Source: CAD feature listing. Evaluate the final solid. Frame: model axes, mm. A direction names the side the tool comes from. Round coordinates to 2 decimals unless told otherwise and drop trailing zeros. Write each loop counter-clockwise with the first axis right and the second up, starting at its lowest first coordinate (ties: lowest second). Pieces come first, ordered by that corner, then holes. Notation, with made-up numbers: (-27.5, 86) -> (-11.5, 86) arc R20 ccw to (-11.5, 99) -> close; hole circle Ø4 at (74, -40). An arc over 180 degrees is marked (long way). Put each result on its own line as item: value.
Autodesk Inventor part; units mm, degrees
ref_plane "YZ Plane" through (0, 0, 0) normal (1, 0, 0) x (0, 1, 0)
ref_plane "XZ Plane" through (0, 0, 0) normal (0, 1, 0) x (-1, 0, 0)
ref_plane "XY Plane" through (0, 0, 0) normal (0, 0, 1) x (1, 0, 0)
sketch "Sketch1" plane through (0, 0, 0) normal (1, 0, 0) x (0, 1, 0)
  line L0 (0, 0) -> (-101.6, 0)
  line L1 (-101.6, 0) -> (-101.6, -25.4)
  line L2 (-101.6, -25.4) -> (0, -25.4)
  line L3 (0, -25.4) -> (0, 0)
  line L4 (-3.175, -3.175) -> (-98.425, -3.175)
  line L5 (-98.425, -3.175) -> (-98.425, -22.225)
  line L6 (-98.425, -22.225) -> (-3.175, -22.225)
  line L7 (-3.175, -22.225) -> (-3.175, -3.175)
  dimension "d0" = 101.6
  dimension "d1" = 25.4
  dimension "d2" = 3.175
extrude "Extrusion1" add sketch "Sketch1" along normal blind 965.2
sketch "Sketch2" plane through (0, -101.6, 0) normal (0, 0, 1) x (1, 0, 0)
  line L0 (909.1795, 114.4192) -> (797.5413, 105.3674)
  arc A0 (797.5413, 105.3674) -> (791.7045, 99.0382) centre (798.0545, 99.0382) ccw
  line L1 (791.7045, 99.0382) -> (791.7045, 2.8001)
  arc A1 (791.7045, 2.8001) -> (797.5413, -3.5291) centre (798.0545, 2.8001) ccw
  line L2 (797.5413, -3.5291) -> (909.1795, -12.5808)
  line L3 (909.1795, -12.5808) -> (910.8305, -12.5808)
  line L4 (910.8305, 114.4192) -> (910.8305, -12.5808)
  line L5 (910.8305, 114.4192) -> (909.1795, 114.4192)
  circle A2 centre (889.5947, 6.3422) radius 2.0447
  circle A3 centre (800.6947, 88.5112) radius 2.0447
  circle A4 centre (889.5947, 104.8942) radius 2.5527
  circle A5 centre (800.6947, 98.5442) radius 2.5527
  circle A6 centre (889.5947, 12.1842) radius 2.5527
  circle A7 centre (800.6947, 82.6692) radius 2.5527
  circle A8 centre (817.7127, 12.1842) radius 5.5562
  circle A9 centre (868.5127, 12.1842) radius 5.5562
  circle A10 centre (817.7127, 89.6542) radius 5.5562
  circle A11 centre (830.5665, 50.9192) radius 11.1061
  circle A12 centre (843.1127, 89.6542) radius 5.5562
  circle A13 centre (868.5127, 89.6542) radius 5.5562
  circle A14 centre (843.1127, 12.1842) radius 5.5562
  circle A15 centre (871.2827, 50.9192) radius 14.2811
  circle A16 centre (800.6947, 19.1692) radius 2.5527
  circle A17 centre (889.5947, 89.6542) radius 2.5527
  circle A18 centre (800.6947, 3.2942) radius 2.5527
  circle A19 centre (889.5947, -3.0558) radius 2.5527
  circle A20 centre (800.6947, 13.3272) radius 2.0447
  circle A21 centre (889.5947, 95.4962) radius 2.0447
  circle A22 centre (800.6947, 3.2942) radius 2.5527
  circle A23 centre (800.6947, 13.3272) radius 2.0447
  circle A24 centre (800.6947, 19.1692) radius 2.5527
  circle A25 centre (800.6947, 82.6692) radius 2.5527
  circle A26 centre (800.6947, 88.5112) radius 2.0447
  circle A27 centre (800.6947, 98.5442) radius 2.5527
  circle A28 centre (830.5665, 50.9192) radius 11.1061
  circle A29 centre (817.7127, 89.6542) radius 5.5563
  circle A30 centre (843.1127, 89.6542) radius 5.5562
  circle A31 centre (868.5127, 89.6542) radius 5.5562
  circle A32 centre (871.2827, 50.9192) radius 14.2811
  circle A33 centre (868.5127, 12.1842) radius 5.5562
  circle A34 centre (843.1127, 12.1842) radius 5.5562
  circle A35 centre (817.7127, 12.1842) radius 5.5562
  circle A36 centre (889.5947, 89.6542) radius 2.5527
  circle A37 centre (889.5947, 95.4962) radius 2.0447
  circle A38 centre (889.5947, 104.8942) radius 2.5527
  circle A39 centre (889.5947, 12.1842) radius 2.5527
  circle A40 centre (889.5947, 6.3422) radius 2.0447
  circle A41 centre (889.5947, -3.0558) radius 2.5527
  point P0 (0, 101.6)
extrude "Extrusion2" cut sketch "Sketch2" against normal blind 25.4 contours A2 | A3 | A4 | A5 | A6 | A7 | A8 | A9 | A10 | A11 | A12 | A13 | A14 | A15 | A16 | A17 | A18 | A19 | A20 | A21
sketch "Sketch3" plane through (0, -101.6, 0) normal (0, 0, 1) x (1, 0, 0)
  line L0 (190.5, -13.3248) -> (181.4483, 98.3133)
  arc A0 (181.4483, 98.3133) -> (175.119, 104.1502) centre (175.119, 97.8002) ccw
  line L1 (175.119, 104.1502) -> (78.881, 104.1502)
  arc A1 (78.881, 104.1502) -> (72.5517, 98.3133) centre (78.881, 97.8002) ccw
  line L2 (72.5517, 98.3133) -> (63.5, -13.3248)
  line L3 (63.5, -13.3248) -> (63.5, -14.9758)
  line L4 (190.5, -14.9758) -> (63.5, -14.9758)
  line L5 (190.5, -14.9758) -> (190.5, -13.3248)
  circle A2 centre (82.423, 6.2599) radius 2.0447
  circle A3 centre (164.592, 95.1599) radius 2.0447
  circle A4 centre (180.975, 6.2599) radius 2.5527
  circle A5 centre (174.625, 95.1599) radius 2.5527
  circle A6 centre (88.265, 6.2599) radius 2.5527
  circle A7 centre (158.75, 95.1599) radius 2.5527
  circle A8 centre (88.265, 78.1419) radius 5.5562
  circle A9 centre (88.265, 27.3419) radius 5.5562
  circle A10 centre (165.735, 78.1419) radius 5.5562
  circle A11 centre (127, 65.2882) radius 11.1061
  circle A12 centre (165.735, 52.7419) radius 5.5562
  circle A13 centre (165.735, 27.3419) radius 5.5562
  circle A14 centre (88.265, 52.7419) radius 5.5562
  circle A15 centre (127, 24.572) radius 14.2811
  circle A16 centre (95.25, 95.1599) radius 2.5527
  circle A17 centre (165.735, 6.2599) radius 2.5527
  circle A18 centre (79.375, 95.1599) radius 2.5527
  circle A19 centre (73.025, 6.2599) radius 2.5527
  circle A20 centre (89.408, 95.1599) radius 2.0447
  circle A21 centre (171.577, 6.2599) radius 2.0447
  circle A22 centre (79.375, 95.1599) radius 2.5527
  circle A23 centre (89.408, 95.1599) radius 2.0447
  circle A24 centre (95.25, 95.1599) radius 2.5527
  circle A25 centre (88.265, 78.1419) radius 5.5562
  circle A26 centre (127, 65.2882) radius 11.1061
  circle A27 centre (88.265, 52.7419) radius 5.5562
  circle A28 centre (88.265, 27.3419) radius 5.5562
  circle A29 centre (88.265, 6.2599) radius 2.5527
  circle A30 centre (82.423, 6.2599) radius 2.0447
  circle A31 centre (73.025, 6.2599) radius 2.5527
  circle A32 centre (127, 24.572) radius 14.2811
  circle A33 centre (165.735, 27.3419) radius 5.5562
  circle A34 centre (165.735, 6.2599) radius 2.5527
  circle A35 centre (171.577, 6.2599) radius 2.0447
  circle A36 centre (180.975, 6.2599) radius 2.5527
  circle A37 centre (165.735, 52.7419) radius 5.5563
  circle A38 centre (165.735, 78.1419) radius 5.5563
  circle A39 centre (164.592, 95.1599) radius 2.0447
  circle A40 centre (158.75, 95.1599) radius 2.5527
  circle A41 centre (174.625, 95.1599) radius 2.5527
  point P0 (0, 101.6)
extrude "Extrusion3" cut sketch "Sketch3" against normal blind 25.4 contours A2 | A3 | A4 | A5 | A6 | A7 | A8 | A9 | A10 | A11 | A12 | A13 | A14 | A15 | A16 | A17 | A18 | A19 | A20 | A21
properties part number "4x1 boxbeam lengths"
Q1. Draft query along Y for faces 1 (the cylindrical face through (140.19, -82.5, -23.79)), 2 (the flat face through (965.2, -55, -23)), 3 (the flat face through (476, 0, -13)). Return one class per face: +Y half, -Y half, draft (parallel to the pull), parting line (faces both ways), or undercut.
Ans:
face 1: undercut
face 2: draft
face 3: +Y half
Q2. Material intervals for line 1 (Z direction, x = 836, y = -5.5) (3 decimals); line 2 (Y direction, x = 769.5, z = -3.75) (3 decimals); line 3 (X direction, y = -41.5, z = -1.75), sorted ascending. Write a range as [from, to].
Ans:
line 1: z = [-25.4, -22.225], [-3.175, 0]
line 2: y = [-101.6, -98.425], [-3.175, 0]
line 3: x = [0, 117.18], [136.82, 824.32], [836.82, 860.34], [882.22, 965.2]
Q3. Cut plane B-B on x = 127. Output: boundary loops of the cut face in (y, z) (3 decimals), and give its area (3 significant figures).
Ans:
outline: (-101.6, -25.4) -> (-91.309, -25.4) -> (-91.309, -22.225) -> (-98.425, -22.225) -> (-98.425, -3.175) -> (-91.309, -3.175) -> (-91.309, 0) -> (-101.6, 0) -> close; (-62.747, -25.4) -> (-47.418, -25.4) -> (-47.418, -22.225) -> (-62.747, -22.225) -> close; (-62.747, -3.175) -> (-47.418, -3.175) -> (-47.418, 0) -> (-62.747, 0) -> close; (-25.206, -25.4) -> (0, -25.4) -> (0, 0) -> (-25.206, 0) -> (-25.206, -3.175) -> (-3.175, -3.175) -> (-3.175, -22.225) -> (-25.206, -22.225) -> close
area: 444 mm^2
Q4. Reachability of faces 4 (the flat face through (883, -3.175, -13)), 5 (the cylindrical face through (140.19, -82.5, -1.57)) from +Z, -Z, +X, -X, +Y, -Y: full face, straight path, thin tool, end or side. Return the list, or none.
Ans:
face 4: +X, -X
face 5: +Z, -Z
Q5. Cut plane A-A on z = -8. Output: boundary loops of the cut face in (x, y) (3 decimals).
Ans:
outline: (0, -101.6) -> (965.2, -101.6) -> (965.2, -98.425) -> (803.245, -98.425) arc R2.553 cw to (798.145, -98.425) -> (0, -98.425) -> close; (0, -3.175) -> (798.145, -3.175) arc R2.553 cw (long way) to (803.245, -3.175) -> (965.2, -3.175) -> (965.2, 0) -> (0, 0) -> close
Q6. Cut plane C-C on x = 422.5. Output: boundary loops of the cut face in (y, z) (3 decimals), and give its area (3 significant figures).
Ans:
outline: (-101.6, -25.4) -> (0, -25.4) -> (0, 0) -> (-101.6, 0) -> close; hole (-98.425, -22.225) -> (-3.175, -22.225) -> (-3.175, -3.175) -> (-98.425, -3.175) -> close
area: 766 mm^2
